from build123d import *

# Parameters (mm, degrees)
CYLINDER1272_R     = 0.8
CYLINDER1272_DEPTH = 10
CYLINDER1273_W     = 55
CYLINDER1273_H     = 60
CYLINDER1273_ANGLE = 80
BOX540_W           = 10
BOX540_H           = 20
BOX540_DEPTH       = 6
BOX539_W           = 5
BOX539_H           = 20
BOX539_DEPTH       = 6
CHAMFER034_SIZE2   = 8
CHAMFER034_SIZE    = 3
CHAMFER035_SIZE2   = 2
CHAMFER035_SIZE    = 11


with BuildPart() as cylinder1443:
    # Cylinder1272 → Cylinder1272 (new body)
    with BuildSketch(Plane(origin=(436.5, 89.5, 42.3), x_dir=(1, 0, 0), z_dir=(0, 0, 1))):
        Circle(CYLINDER1272_R)
    extrude(amount=CYLINDER1272_DEPTH)


with BuildPart() as cylinder1273:
    # Cylinder1273 → Cylinder1273 (revolve)
    with BuildSketch(Plane(origin=(432, 85, 100), x_dir=(0, 0, -1), z_dir=(0, -1, 0))):
        with Locations((27.5, 30)):
            Rectangle(CYLINDER1273_W, CYLINDER1273_H)
    revolve(axis=Axis((432, 85, 100), (1, 0, 0)), revolution_arc=CYLINDER1273_ANGLE)


with BuildPart() as fusion248002050161:
    # Box540 → Box540 (new body)
    with BuildSketch(Plane(origin=(434, 65, 44.75), x_dir=(1, 0, 0), z_dir=(0, 0, 1))):
        with Locations((5, 10)):
            Rectangle(BOX540_W, BOX540_H)
    extrude(amount=BOX540_DEPTH)

    # Fusion248002050161: union Cylinder1273
    add(cylinder1273.part)


with BuildPart() as bucket_tooth:
    # Box539 → Box539 (new body)
    with BuildSketch(Plane(origin=(434, 78, 42), x_dir=(1, 0, 0), z_dir=(0, 0, 1))):
        with Locations((2.5, 10)):
            Rectangle(BOX539_W, BOX539_H)
    extrude(amount=BOX539_DEPTH)

    # Cut014288: cut Fusion248002050161
    add(fusion248002050161.part, mode=Mode.SUBTRACT)

    # Chamfer034
    chamfer034_edges = [bucket_tooth.edges().sort_by_distance(p)[0] for p in [
        (436.5, 98, 42),
    ]]
    chamfer034_side = bucket_tooth.faces().sort_by_distance((436.5, 98, 44.279222))[0]
    chamfer(chamfer034_edges, length=CHAMFER034_SIZE, length2=CHAMFER034_SIZE2, reference=chamfer034_side)

    # Chamfer035
    chamfer035_edges = [bucket_tooth.edges().sort_by_distance(p)[0] for p in [
        (436.5, 78, 42),
    ]]
    chamfer035_side = bucket_tooth.faces().sort_by_distance((436.5, 84, 42))[0]
    chamfer(chamfer035_edges, length=CHAMFER035_SIZE, length2=CHAMFER035_SIZE2, reference=chamfer035_side)

    # Cut014289: cut Cylinder1443
    add(cylinder1443.part, mode=Mode.SUBTRACT)


solid = bucket_tooth.part
Source: CAD feature listing. Evaluate the final solid. Frame: model axes, mm. A direction names the side the tool comes from. Round coordinates to 2 decimals unless told otherwise and drop trailing zeros. Loops run counter-clockwise (first coordinate to the right, second up) from the corner with the lowest first, then second, coordinate; pieces in that order, holes last. Notation, with made-up numbers: (-17, 51.5) -> (16, 51.5) arc R18 cw to (16, 67.5) -> close; hole circle Ø8 at (53, 32). An arc over 180 degrees is marked (long way). Answer as a JSON object with one key per item and string values. Group by question number.
Q1. Section query C-C (y = 89.5). Output: boundary loops of the cut face in (x, z), plus the area to 3 significant figures.
Q2. Ray query, line 1 (X direction, y = 89.5, z = 44.45); line 2 (Z direction, x = 436.35, y = 89.25); line 3 (Z direction, x = 434.5, y = 85.5). Return the intervals inside material, ascending. Write a range as from..to.
Q3. Access query for faces 1 (the flat face through (436, 82, 44.75)), 2 (the flat face through (434, 90, 44)), 3 (the cylindrical face through (435.7, 89.5, 43.8)). Directions: +Z, -Z, +X, -X, +Y, -Y. A direction counts if a zero-diameter tool reaches every point of the face in a straight line with its end or side. Return the directions, or none.
Q4. Section query D-D (z = 43.8). Output: boundary loops of the cut face in (x, y), plus the area to 3 significant figures.
Q5. Section query B-B (x = 438.4). Output: boundary loops of the cut face in (y, z).
Q6. Contact query for flat-ended pins moving along their axis: P1, Ø2, axis at x = 438.5, y = 83, coming from the +Z side; P2, Ø1.3, axis at x = 436.5, y = 89.5, coming from the +Z side. Output: stop coordinate, or through.
Q7. Mould query, pull axis Y, two halves, no side actions, for faces 4 (the flat face through (436, 98, 46)), 5 (the flat face through (436.5, 89.5, 42.3)), 6 (the flat face through (436.465, 83.423, 43.014)). Classes: pulls with the +Y half, pulls with the -Y half, needs draft (parallel to the pull), parting line crosses it, or undercut.
Q8. Section query A-A (z = 44.55). Output: boundary loops of the cut face in (x, y), plus the area to 3 significant figures.
Completed:
{
 "1": {"outline": "(434, 42) -> (439, 42) -> (439, 45.18) -> (437.3, 45.18) -> (437.3, 42.3) -> (435.7, 42.3) -> (435.7, 45.18) -> (434, 45.18) -> close", "area": "11.3 mm²"},
 "2": {"line 1": "434..435.7, 437.3..439", "line 2": "42..42.3", "line 3": "42.64..45"},
 "3": {"face 1": "+Z, +X, -X, -Y", "face 2": "+Z, -Z, -X, +Y, -Y", "face 3": "+Z"},
 "4": {"outline": "(434, 79.1) -> (439, 79.1) -> (439, 94.8) -> (434, 94.8) -> close; hole circle Ø1.6 at (436.5, 89.5)", "area": "76.5 mm²"},
 "5": {"outline": "(78, 44) -> (89, 42) -> (90, 42) -> (98, 45) -> (98, 46.56) arc R55 cw to (85, 45) -> (85, 44.75) -> (78, 44.75) -> close"},
 "6": {"P1": "z = 44.75", "P2": "z = 42.3"},
 "7": {"face 4": "pulls with the +Y half", "face 5": "undercut", "face 6": "pulls with the -Y half"},
 "8": {"outline": "(434, 78) -> (439, 78) -> (439, 96.8) -> (434, 96.8) -> close; hole circle Ø1.6 at (436.5, 89.5)", "area": "92.0 mm²"}
}
